from build123d import *

# Parameters (mm, degrees)
F1_DEPTH = 2
F2_R     = 4
F3_DEPTH = 19
F4_R     = 1.25
F5_DEPTH = 21.001
F6_R     = 1.25
F7_DEPTH = 21.001
F8_R     = 26


with BuildPart() as f1:
    # F0 (on Top) → F1 (new body)
    with BuildSketch(Plane.XY):
        with BuildLine():
            ThreePointArc((-17.5, 19), (-21.5, 15), (-25.5, 19))
            Line((-25.5, 19), (-25.5, -23))
            Line((-25.5, -23), (21.5, -23))
            ThreePointArc((21.5, -23), (17.737893, -17.641123), (24.056121, -15.923274))
            Line((24.056121, -15.923274), (-18.851111, 21.99723))
            ThreePointArc((-18.851111, 21.99723), (-17.853388, 20.643844), (-17.5, 19))
        make_face()
        with BuildLine():
            ThreePointArc((-18.851111, 21.99723), (-23.143844, 22.646612), (-25.5, 19))
            ThreePointArc((-25.5, 19), (-21.5, 15), (-17.5, 19))
            ThreePointArc((-17.5, 19), (-17.853388, 20.643844), (-18.851111, 21.99723))
        make_face()
        with BuildLine():
            ThreePointArc((24.056121, -15.923274), (17.737893, -17.641123), (21.5, -23))
            ThreePointArc((21.5, -23), (24.328427, -21.828427), (25.5, -19))
            ThreePointArc((25.5, -19), (25.121083, -17.30066), (24.056121, -15.923274))
        make_face()
    extrude(amount=F1_DEPTH)

    # F2 (on face) → F3 (join)
    with BuildSketch(Plane.XY.offset(2)):
        with Locations((-21.5, 19)):
            Circle(F2_R)
        with Locations((21.5, -19)):
            Circle(F2_R)
    extrude(amount=F3_DEPTH)

    # F4 (on face) → F5 (cut, through all)
    with BuildSketch(Plane.XY.offset(21)):
        with Locations((-21.5, 19)):
            Circle(F4_R)
    extrude(amount=-F5_DEPTH, mode=Mode.SUBTRACT)

    # F6 (on face) → F7 (cut, through all)
    with BuildSketch(Plane.XY.offset(21)):
        with Locations((21.5, -19)):
            Circle(F6_R)
    extrude(amount=-F7_DEPTH, mode=Mode.SUBTRACT)

    # F8
    f8_edges = [f1.edges().sort_by_distance(p)[0] for p in [
        (-25.5, -23, 1),
    ]]
    fillet(f8_edges, radius=F8_R)


solid = f1.part
Input: part model. Units: mm. Frame: model coordinates. Coordinates: 2 decimals unless noted, no trailing zeros. Loops run counter-clockwise (first coordinate to the right, second up) from the corner with the lowest first, then second, coordinate; pieces in that order, holes last. Notation, with made-up numbers: (51.5, 27) -> (110.5, 27) arc R19 cw to (110.5, 49) -> close; hole circle Ø5 at (63.25, 80). An arc over 180 degrees is marked (long way). One line per item, written item: value.
(1) Cut plane A-A (x = -21.5). Output: boundary loops of the cut face in (y, z).
Answer below:
outline: (-10.86, 0) -> (17.75, 0) -> (17.75, 21) -> (15, 21) -> (15, 2) -> (-10.86, 2) -> close; (20.25, 0) -> (23, 0) -> (23, 21) -> (20.25, 21) -> close
(2) Draft query along X for faces 1 (the face through (23, -19, 21)), 2 (the face through (22.655, -19.479, 10.647)), 3 (the face through (-25.5, 11, 1)). Return one class per face: pulls with the +X half, pulls with the -X half, needs draft (parallel to the pull), parting line crosses it, or undercut.
Answer below:
face 1: needs draft
face 2: undercut
face 3: pulls with the -X half
(3) Cut plane C-C (y = -17). Output: boundary loops of the cut face in (x, z), then the cut area to 3 significant figures.
Answer below:
outline: (-16.11, 0) -> (24.96, 0) -> (24.96, 21) -> (18.04, 21) -> (18.04, 2) -> (-16.11, 2) -> close
area: 214 mm2
(4) Cut plane B-B (z = 8.5). Output: boundary loops of the cut face in (x, y).
Answer below:
outline: circle Ø8 at (-21.5, 19); circle Ø8 at (21.5, -19); hole circle Ø2.5 at (-21.5, 19); hole circle Ø2.5 at (21.5, -19)
(5) Ray query, line 1 along Y through (x, z) = (21.5, 11.5); line 2 along Y through (x, z) = (-21.5, 9.25); line 3 along Z through (x, y) = (-23, -2.5). Return the intervals inside material, ascending.
Answer below:
line 1: y = -23 to -20.25, -17.75 to -15
line 2: y = 15 to 17.75, 20.25 to 23
line 3: z = 0 to 2
(6) Cut plane D-D (x = 5). Output: boundary loops of the cut face in (y, z), then the cut area to 3 significant figures.
Answer below:
outline: (-23, 0) -> (0.92, 0) -> (0.92, 2) -> (-23, 2) -> close
area: 47.8 mm2
